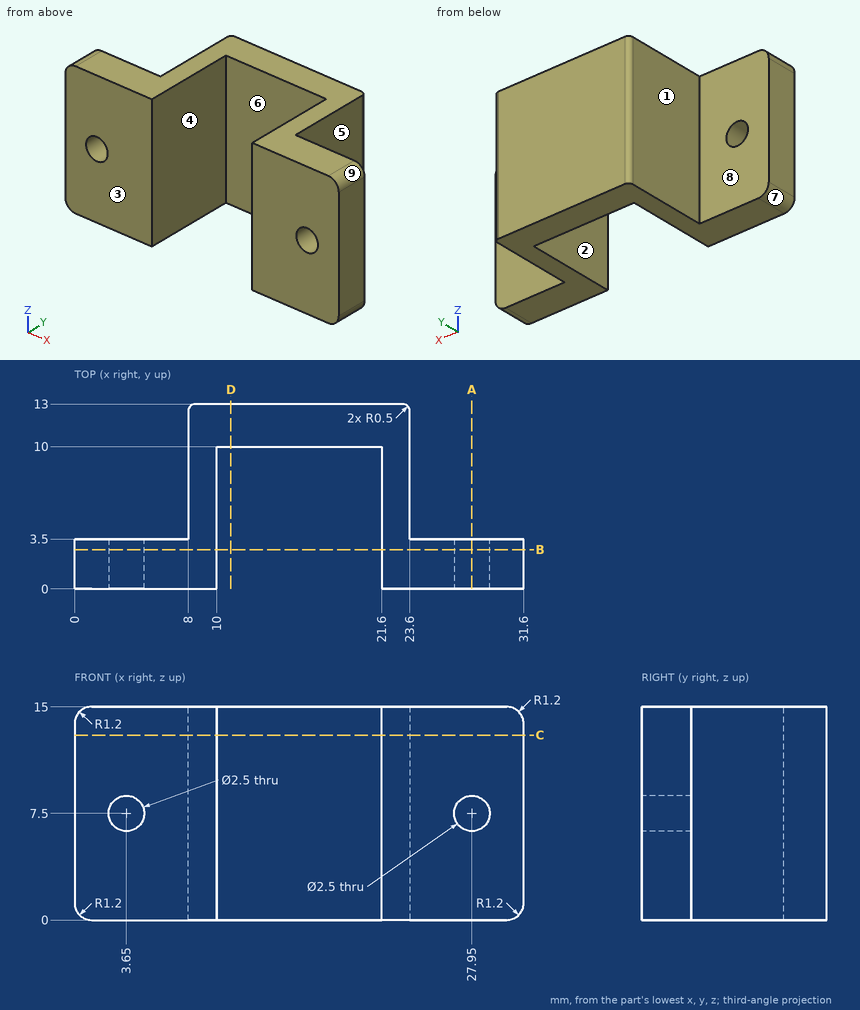
Input: dimensioned drawing with shaded views. Units: mm. Origin: part minimum x, y, z. A direction names the side the tool comes from. Coordinates: 2 decimals unless noted, no trailing zeros. Loops run counter-clockwise (first coordinate to the right, second up) from the corner with the lowest first, then second, coordinate; pieces in that order, holes last. Notation, with made-up numbers: M 30.25,-26.5 L 44.25,-26.5 A29 ccw 44.25,11.5 Z; hole C 4,26 d3. An arc over 180 degrees is marked long. Use a Markdown table: item, result. Add a question column.
Q1. Draft query along X for the marked faces 1, 2, 3 and 4. Return one class per face: pulls with the +X half, pulls with the -X half, needs draft (parallel to the pull), parting line crosses it, or undercut.
Q2. Section query B-B, the plane y = 2.75. Return loops of the section in (x, z), and give its area (3 significant figures).
Q3. Section query A-A, the plane x = 27.95. Return loops of the section in (y, z).
Q4. Access query for the marked faces 5, 6, 7, 8 and 9. Directions: +Z, -Z, +X, -X, +Y, -Y. A direction counts if a zero-diameter tool reaches every point of the face in a straight line with its end or side. Return the directions, or none.
Q5. Section query C-C, the plane z = 13. Return loops of the section in (x, y), and give its area (3 significant figures).
Q6. Material intervals for L1, parallel to X at y = 2.6, z = 7.5; L2, parallel to Z at x = 27.95, y = 2.45; L3, parallel to X at y = 7.5, z = 1.75, sorted ascending.
Q7. First-contact query: pin 1 (2 mm diameter, centred on y = 5, z = 9.5, fed in from -X); pin 2 (6.5 mm diameter, centred on x = 29, z = 4, fed in from +Y). Flat tips, straight axial feed; report the tip coordinate or a pass-through.
Q8. Section query D-D, the plane x = 11. Return loops of the section in (y, z), and give its area (3 significant figures).
Result:
| question | item | result |
|---|---|---|
| 1 | face 1 | pulls with the -X half |
| 1 | face 2 | undercut |
| 1 | face 3 | needs draft |
| 1 | face 4 | undercut |
| 2 | outline | M 0,1.2 A1.2 ccw 1.2,0 L 10,0 L 10,15 L 1.2,15 A1.2 ccw 0,13.8 Z; M 21.6,0 L 30.4,0 A1.2 ccw 31.6,1.2 L 31.6,13.8 A1.2 ccw 30.4,15 L 21.6,15 Z; hole C 3.65,7.5 d2.5; hole C 27.95,7.5 d2.5 |
| 2 | area | 289 mm2 |
| 3 | outline | M 0,0 L 3.5,0 L 3.5,6.25 L 0,6.25 Z; M 0,8.75 L 3.5,8.75 L 3.5,15 L 0,15 Z |
| 4 | face 5 | +Z, -Z, +X, +Y |
| 4 | face 6 | +Z, -Z, -Y |
| 4 | face 7 | -Z, -X, +Y, -Y |
| 4 | face 8 | +Z, -Z, -X, +Y |
| 4 | face 9 | +Z, +X, +Y, -Y |
| 5 | outline | M 0,0 L 10,0 L 10,10 L 21.6,10 L 21.6,0 L 31.6,0 L 31.6,3.5 L 23.6,3.5 L 23.6,12.5 A0.5 ccw 23.1,13 L 8.5,13 A0.5 ccw 8,12.5 L 8,3.5 L 0,3.5 Z |
| 5 | area | 143 mm2 |
| 6 | L1 | x = 0 to 2.4, 4.9 to 10, 21.6 to 26.7, 29.2 to 31.6 |
| 6 | L2 | z = 0 to 6.25, 8.75 to 15 |
| 6 | L3 | x = 8 to 10, 21.6 to 23.6 |
| 7 | pin 1 | stops at x = 8 |
| 7 | pin 2 | stops at y = 3.5 |
| 8 | outline | M 10,0 L 13,0 L 13,15 L 10,15 Z |
| 8 | area | 45.0 mm2 |
